Verification items for this drawing (mm, ordinates from the low corner). A direction names the side the tool comes from. Coordinates: 2 decimals unless noted, no trailing zeros. Write each loop counter-clockwise with the first axis right and the second up, starting at its lowest first coordinate (ties: lowest second). Pieces come first, ordered by that corner, then holes. Notation, with made-up numbers: M 35.25,62.5 L 88.25,62.5 A27 cw 88.25,81.5 Z; hole C -38.5,28.25 d6. An arc over 180 degrees is marked long. Put each result on its own line as item: value. Start each with the question number.
1) Gauge pin test, flat ends, axial feed: pin 1 (3 mm diameter, centred on x = 8.5, y = 8, fed in from -Z); pin 2 (1.5 mm diameter, centred on x = 2, y = 3, fed in from +Z); pin 3 (6 mm diameter, centred on x = 7, y = 1.5, fed in from +Z). Record the tip position at first contact, or that the pin passes through.
2) Cross-section at A-A on z = 11. Record the cut outline in (x, y), plus the area to 3 significant figures.
3) Scan lines: line 1 along Z through (x, y) = (8.75, 1.5); line 2 along Y through (x, z) = (2, 10.25); line 3 along Z through (x, y) = (9.25, 4.75). Record each from-to range of solid material in increasing order.
4) Set-up check for the marked faces 1 and 2: record each of +Z, -Z, +X, -X, +Y, -Y from which the full face is reachable in a straight line by a thin tool's end or side.
5) Mould release check, pull along Y, two halves, no side actions. Record for the marked faces 3, 4 and 5: released by +Y, released by -Y, zero draft, split by the parting line, or undercut.
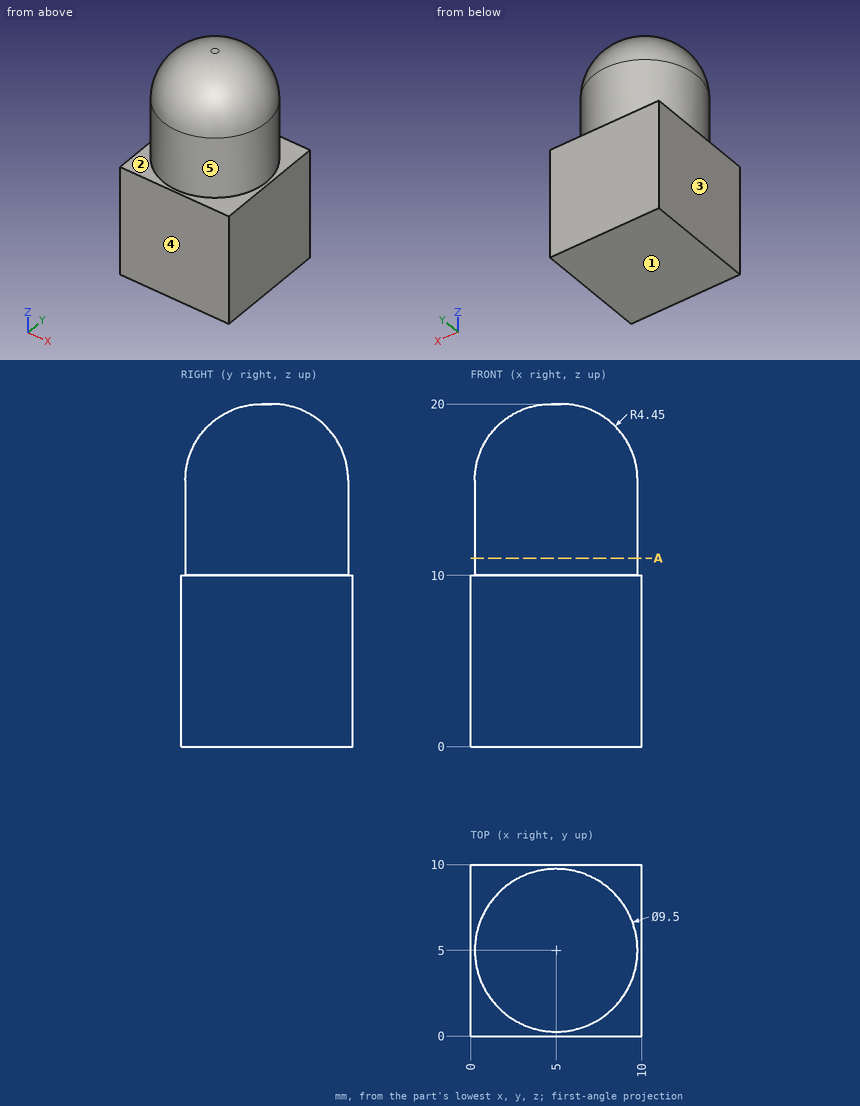
Answer key:
1. pin 1: stops at z = 0
1. pin 2: stops at z = 19.19
1. pin 3: stops at z = 19.94
2. outline: C 5,5 d9.5
2. area: 70.9 mm²
3. line 1: z = 0 to 10
3. line 2: y = 1.32 to 8.68
3. line 3: z = 0 to 17.59
4. face 1: -Z, +X, -X, +Y, -Y
4. face 2: +Z
5. face 3: zero draft
5. face 4: released by -Y
5. face 5: split by the parting line
